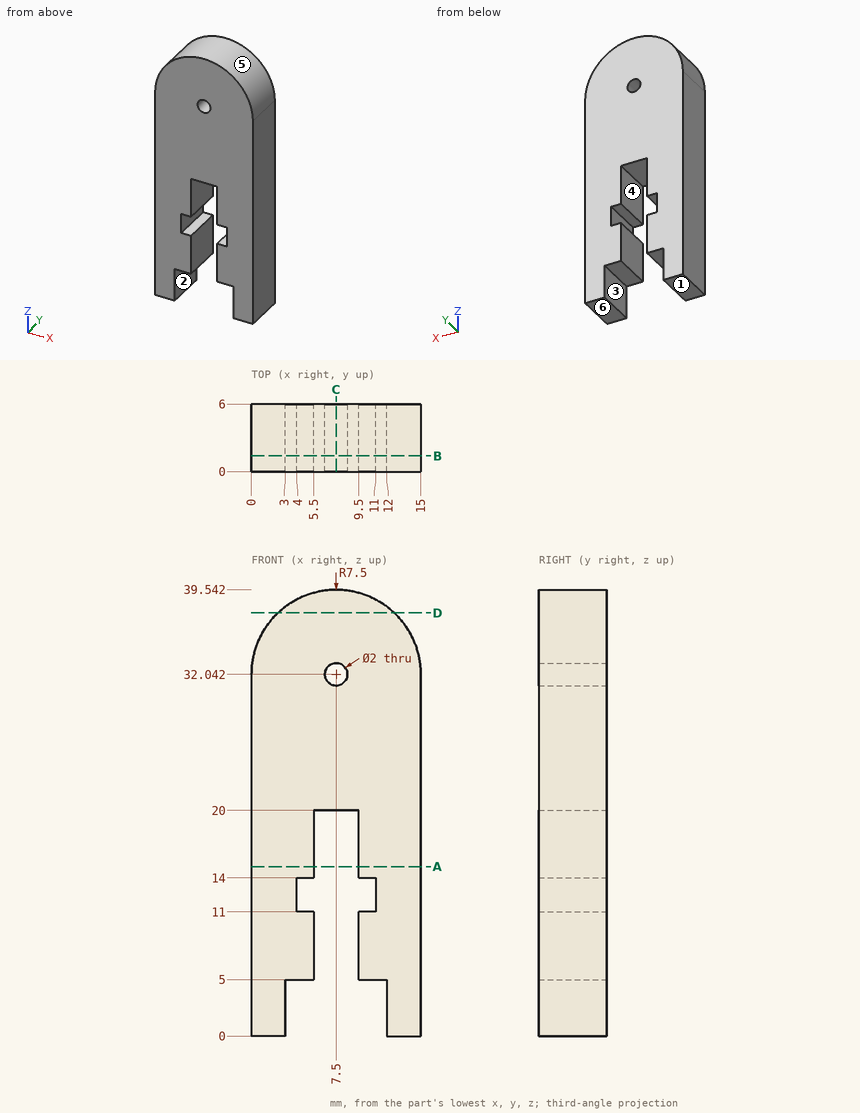
Design review of the part shown in the three views and the two pictorial views. Dimensions are in mm from the part's minimum x, y and z. A direction names the side the tool comes from. Round coordinates to 2 decimals unless told otherwise and drop trailing zeros. Write each loop counter-clockwise with the first axis right and the second up, starting at its lowest first coordinate (ties: lowest second). Pieces come first, ordered by that corner, then holes. Notation, with made-up numbers: (29.25, 78.25) -> (51.25, 78.25) arc R3 cw to (51.25, 83.25) -> close; hole circle Ø6 at (8.25, 6). An arc over 180 degrees is marked (long way). One line per question, with ' | ' between items. Start each with the question number.
1) Add section B-B (y = 1.4). Write out the cut boundary in (x, z).
2) Machinability: for the marked faces 1 and 2, which of the approach directions +Z, -Z, +X, -X, +Y, -Y give a long, thin tool a straight path to every point of the face, cutting with its end or side? Answer none if there is none.
3) Add section D-D (z = 37.5). Write out the cut boundary in (x, y), and give its area (3 significant figures).
4) Add section C-C (x = 7.5). Write out the cut boundary in (y, z).
5) Add section A-A (z = 15). Write out the cut boundary in (x, y), and give its area (3 significant figures).
6) For pin 1 Ø2 at (x, y) = (5.5, 3) entering from -Z; pin 2 Ø1.2 at (x, z) = (7.5, 32.04) entering from +Y; pin 3 Ø1.6 at (x, y) = (10.5, 3.5) entering from +Z; pin 4 Ø1.6 at (x, y) = (5, 2.5) entering from +Z, all flat-tipped, find the tip position at first contact; note any pin that passes through.
7) Mouldability with a two-part tool opening along X and no side actions: class the marked faces 3, 4, 5 and 6 as +X half, -X half, draft (parallel to the pull), parting line (faces both ways), or undercut.
8) Wall thickness on line 1 along X through (y, z) = (3.2, 15.5); line 2 along X through (y, z) = (4.55, 2); line 3 along Z through (x, y) = (7.5, 3.1): over which ranges is each line inside the solid? List them lowest first.
Reported:
1) outline: (0, 0) -> (3, 0) -> (3, 5) -> (5.5, 5) -> (5.5, 11) -> (4, 11) -> (4, 14) -> (5.5, 14) -> (5.5, 20) -> (9.5, 20) -> (9.5, 14) -> (11, 14) -> (11, 11) -> (9.5, 11) -> (9.5, 5) -> (12, 5) -> (12, 0) -> (15, 0) -> (15, 32.04) arc R7.5 ccw to (0, 32.04) -> close; hole circle Ø2 at (7.5, 32.04)
2) face 1: -Z, +X, -X, +Y, -Y | face 2: -Z, +Y, -Y
3) outline: (2.36, 0) -> (12.64, 0) -> (12.64, 6) -> (2.36, 6) -> close | area: 61.7 mm²
4) outline: (0, 20) -> (6, 20) -> (6, 31.04) -> (0, 31.04) -> close; (0, 33.04) -> (6, 33.04) -> (6, 39.54) -> (0, 39.54) -> close
5) outline: (0, 0) -> (5.5, 0) -> (5.5, 6) -> (0, 6) -> close; (9.5, 0) -> (15, 0) -> (15, 6) -> (9.5, 6) -> close | area: 66.0 mm²
6) pin 1: stops at z = 5 | pin 2: passes through | pin 3: stops at z = 39.21 | pin 4: stops at z = 39.35
7) face 3: undercut | face 4: undercut | face 5: parting line | face 6: draft
8) line 1: x = 0 to 5.5, 9.5 to 15 | line 2: x = 0 to 3, 12 to 15 | line 3: z = 20 to 31.04, 33.04 to 39.54
